Design review of the part built by this model. Coordinates are the model's own, in mm. A direction names the side the tool comes from. Give positions to 0.01 mm unless a question says otherwise; leave off trailing zeros. Loops run counter-clockwise (first coordinate to the right, second up) from the corner with the lowest first, then second, coordinate; pieces in that order, holes last. Notation, with made-up numbers: (11.5, -25.5) -> (50.5, -25.5) arc R17 ccw to (50.5, -10.5) -> close; hole circle Ø5 at (-6.5, 79.25). An arc over 180 degrees is marked (long way). Use a Markdown table: item, result. Add a question column.
1. For pin 1 Ø8 at (x, z) = (-9.5, -14) entering from -Y; pin 2 Ø3 at (x, y) = (6.5, -1.5) entering from -Z; pin 3 Ø10 at (x, y) = (9.5, 4.5) entering from +Z, all flat-tipped, find the tip position at first contact; note any pin that passes through.
2. Add section D-D (z = -19.5). State the section outline as (x, y) points.
3. Draft analysis for pull direction X (two halves, no side actions). For faces 1 (the flat face through (-12.6, 0, 1)), 2 (the flat face through (-6, 0, -17)), 3 (the cylindrical face through (0.14, -11.7, 2.22)), state which applies: pulls with the +X half, pulls with the -X half, needs draft (parallel to the pull), parting line crosses it, or undercut.
4. Add section A-A (z = -7.5). State the section outline as (x, y) points, and give its area (3 significant figures).
5. Add section B-B (x = -4.5). State the section outline as (y, z) points.
6. For faces 4 (the flat face through (-12, 0, 0)), 5 (the flat face through (0, 12.5, 1)), 6 (the flat face through (0.65, 0, -24)), 7 (the flat face through (-0.65, 0, -24)), 8 (the flat face through (0, -15.7, 1)), list the 3-axis set-ups (+Z, -Z, +X, -X, +Y, -Y) from which the entire face can be reached by the end or side of a thin tool; tool diameter is ignored.
7. To check wall thickness, follow line 1 (X direction, y = 10, z = 1); line 2 (X direction, y = 6.5, z = -30); line 3 (Z direction, x = -11.25, y = -9). State the ranges of each line that lie inside material, in increasing order.
Autodesk Inventor part; units mm, degrees
ref_plane "Work Plane1" through (0, -12.5, 2) normal (-1, 0, 0) x (0, 0, 1)
ref_plane "YZ Plane" through (0, 0, 0) normal (1, 0, 0) x (0, 1, 0)
ref_plane "XZ Plane" through (0, 0, 0) normal (0, 1, 0) x (-1, 0, 0)
sketch "Sketch1" plane through (0, 0, 0) normal (0, 0, 1) x (1, 0, 0)
  point P0 (0, 0)
sketch "Sketch2" plane through (0, 0, 0) normal (0, 0, 1) x (1, 0, 0)
  line L0 (-12.6, -15.7) -> (12.6, -15.7)
  line L1 (12.6, -15.7) -> (12.6, 15.7)
  line L2 (12.6, 15.7) -> (-12.6, 15.7)
  line L3 (-12.6, 15.7) -> (-12.6, -15.7)
  line L4 (-12.6, -15.7) -> (12.6, 15.7) construction
  line L5 (12.6, -15.7) -> (-12.6, 15.7) construction
  point P0 (0, 0)
  dimension "d0" = 25.2
  dimension "d1" = 31.4
extrude "Extrusion1" add sketch "Sketch2" along normal blind 2
sketch "Sketch3" plane through (0, 0, 0) normal (0, 0, -1) x (-1, 0, 0)
  line L0 (-10.9, -14.5) -> (10.9, -14.5)
  line L1 (10.9, -14.5) -> (10.9, 14.5)
  line L2 (10.9, 14.5) -> (-10.9, 14.5)
  line L3 (-10.9, 14.5) -> (-10.9, -14.5)
  line L4 (-10.9, -14.5) -> (10.9, 14.5) construction
  line L5 (10.9, -14.5) -> (-10.9, 14.5) construction
  point P0 (0, 0)
  dimension "d4" = 21.8
  dimension "d5" = 29
extrude "Extrusion2" add sketch "Sketch3" along normal blind 17
sketch "Sketch4" plane through (0, 0, -17) normal (0, 0, -1) x (-1, 0, 0)
  line L0 (-0.65, 14.5) -> (0.65, 14.5)
  line L1 (0.65, 14.5) -> (0.65, -14.5)
  line L2 (0.65, -14.5) -> (-0.65, -14.5)
  line L3 (-0.65, -14.5) -> (-0.65, 14.5)
  line L4 (-0.65, 14.5) -> (0.65, -14.5) construction
  line L5 (0.65, 14.5) -> (-0.65, -14.5) construction
  line L6 (-10.9, -14.5) -> (10.9, -14.5)
  point P0 (0, 0)
  point P1 (0, -14.5)
  dimension "d8" = 1.3
extrude "Extrusion3" add sketch "Sketch4" along normal blind 15
sketch "Sketch5" plane through (0, 0, 2) normal (0, 0, 1) x (1, 0, 0)
  line L0 (-10, -12.5) -> (10, -12.5)
  line L1 (10, -12.5) -> (10, 12.5)
  line L2 (10, 12.5) -> (-10, 12.5)
  line L3 (-10, 12.5) -> (-10, -12.5)
  line L4 (-10, -12.5) -> (10, 12.5) construction
  line L5 (10, -12.5) -> (-10, 12.5) construction
  point P0 (0, 0)
  dimension "d11" = 20
  dimension "d12" = 25
extrude "Extrusion4" cut sketch "Sketch5" against normal blind 2
ref_plane "Work Plane1" through (0, -12.5, 2) normal (-1, 0, 0) x (0, 0, 1)
sketch "Sketch6" plane through (0, -12.5, 2) normal (-1, 0, 0) x (0, 0, 1)
  arc A0 (3.3287, 21.9761) -> (0.5045, 1.4881) centre (83.3994, 0.5) ccw
  line L0 (2.6334, 23.1979) -> (-2, 24.5)
  line L1 (-0.4954, 0.5) -> (-2, 0.5)
  line L2 (-2, 0) -> (-2, 25)
  arc A1 (3.3287, 21.9761) -> (2.6334, 23.1979) centre (2.3628, 22.2352) ccw
  arc A2 (-0.4954, 0.5) -> (0.5045, 1.4881) centre (-0.4954, 1.5) ccw
  line L3 (-2, 0.5) -> (-2, 24.5)
  point P0 (-2, 12.5)
  point P1 (3.5903, 22.9289)
  point P2 (0.4986, 0.5)
  dimension "d15" = 0.5
  dimension "d16" = 0.5
  dimension "d17" = 2.4986
  dimension "d18" = 5.5903
  dimension "d19" = 1
extrude "Extrusion5" add sketch "Sketch6" along normal mid plane 19.5
fillet "Fillet1" radius 0.2 33 edges at (-12.6, 0, 2) (0, -15.7, 2) (0, -15.7, 0) (-12.6, -15.7, 1) (-12.6, 0, 0) (12.6, 0, 2) (12.6, 0, 0) (0, 15.7, 2) (0, 15.7, 0) (-12.6, 15.7, 1) (12.6, -15.7, 1) (12.6, 15.7, 1) (10.9, -14.5, -8.5) (10.9, 14.5, -8.5) (0.65, 14.5, -24.5) (5.775, -14.5, -17) (0.65, -14.5, -24.5) (-0.65, -14.5, -24.5) (-5.775, -14.5, -17) (-10.9, -14.5, -8.5) (10.9, 0, -17) (5.775, 14.5, -17) (-5.775, 14.5, -17) (-0.65, 0, -32) (0.65, 0, -32) (0, 14.5, -32) (0, -14.5, -32) (-10.9, 0, -17) (-10.9, 14.5, -8.5) (-10.9, 0, 0) (0, -14.5, 0) (10.9, 0, 0) (0, 14.5, 0)
properties part number "On_Off_Switch"
Taken from the geometry:
| question | item | result |
|---|---|---|
| 1 | pin 1 | stops at y = -14.5 |
| 1 | pin 2 | stops at z = -17 |
| 1 | pin 3 | stops at z = 5.33 |
| 2 | outline | (-0.65, -14.3) arc R0.2 ccw to (-0.45, -14.5) -> (0.45, -14.5) arc R0.2 ccw to (0.65, -14.3) -> (0.65, 14.3) arc R0.2 ccw to (0.45, 14.5) -> (-0.65, 14.5) -> close |
| 3 | face 1 | pulls with the -X half |
| 3 | face 2 | needs draft |
| 3 | face 3 | undercut |
| 4 | outline | (-10.9, -14.3) arc R0.2 ccw to (-10.7, -14.5) -> (10.7, -14.5) arc R0.2 ccw to (10.9, -14.3) -> (10.9, 14.3) arc R0.2 ccw to (10.7, 14.5) -> (-10.7, 14.5) arc R0.2 ccw to (-10.9, 14.3) -> close |
| 4 | area | 632 mm^2 |
| 5 | outline | (-15.7, 0.2) arc R0.2 ccw to (-15.5, 0) -> (-14.7, 0) arc R0.2 cw to (-14.5, -0.2) -> (-14.5, -16.8) arc R0.2 ccw to (-14.3, -17) -> (14.3, -17) arc R0.2 ccw to (14.5, -16.8) -> (14.5, -0.2) arc R0.2 cw to (14.7, 0) -> (15.5, 0) arc R0.2 ccw to (15.7, 0.2) -> (15.7, 1.8) arc R0.2 ccw to (15.5, 2) -> (12.5, 2) -> (12.5, 0) -> (12, 0) -> (10.7, 4.63) arc R1 ccw to (9.48, 5.33) arc R82.9 cw to (-11.01, 2.5) arc R1 ccw to (-12, 1.5) -> (-12, 0) -> (-12.5, 0) -> (-12.5, 2) -> (-15.5, 2) arc R0.2 ccw to (-15.7, 1.8) -> close |
| 6 | face 4 | -Z |
| 6 | face 5 | +Z |
| 6 | face 6 | -Z, +X, +Y, -Y |
| 6 | face 7 | -Z, -X, +Y, -Y |
| 6 | face 8 | +Z, -Z, +X, -X, -Y |
| 7 | line 1 | x = -12.6 to -10, -9.75 to 9.75, 10 to 12.6 |
| 7 | line 2 | x = -0.65 to 0.65 |
| 7 | line 3 | z = 0 to 2 |
